```python
from build123d import *

# Parameters (mm, degrees)
SKETCH2_R           = 30
BOSS_EXTRUDE1_DEPTH = 15
SKETCH3_R           = 2.25
CUT_EXTRUDE1_DEPTH  = 9
FILLET1_R           = 1.5
CUT_EXTRUDE2_DEPTH  = 1
SKETCH5_W           = 5
SKETCH5_H           = 19.75
CUT_EXTRUDE3_DEPTH  = 10
CIRPATTERN1_COUNT   = 6


with BuildPart() as part:
    # Sketch2 → Boss-Extrude1 (new body)
    with BuildSketch(Plane(origin=(0, 0, 0), x_dir=(1, 0, 0), z_dir=(0, 1, 0))):
        with Locations(Location((0, 0, 0), (0, 0, 270))):
            Circle(SKETCH2_R)
    extrude(amount=BOSS_EXTRUDE1_DEPTH)

    # Sketch3 → Cut-Extrude1 (cut)
    with BuildSketch(Plane(origin=(0, 15, 0), x_dir=(1, 0, 0), z_dir=(0, 1, 0))):
        with Locations(Location((0, 0, 0), (0, 0, 270))):
            Circle(SKETCH3_R)
    extrude(amount=-CUT_EXTRUDE1_DEPTH, mode=Mode.SUBTRACT)

    # Fillet1
    fillet1_edges = [part.edges().sort_by_distance(p)[0] for p in [
        (0, 0, -30),
        (0, 15, -30),
        (0, 15, -2.25),
    ]]
    fillet(fillet1_edges, radius=FILLET1_R)

    # Sketch4 → Cut-Extrude2 (cut)
    with BuildSketch(Plane.XZ):
        Polygon((-0.5, 24.5), (-0.5, -27.5), (0.5, -27.5), (0.5, 24.5), (3, 24.5), (0, 27.5), (-3, 24.5), align=None)
    extrude(amount=-CUT_EXTRUDE2_DEPTH, mode=Mode.SUBTRACT)

    # Sketch5 → Cut-Extrude3 (cut)
    with BuildSketch(Plane(origin=(0, 15, 0), x_dir=(1, 0, 0), z_dir=(0, 1, 0))):
        with Locations((0, 16.125)):
            Rectangle(SKETCH5_W, SKETCH5_H)
    cut_extrude3 = extrude(amount=-CUT_EXTRUDE3_DEPTH, mode=Mode.SUBTRACT)

    # CirPattern1: Cut-Extrude3 ×6 about axis
    cirpattern1_axis = Axis((0, 0, 0), (0, 1, 0))
    for i in range(1, CIRPATTERN1_COUNT):
        add(cut_extrude3.rotate(cirpattern1_axis, i * 360 / CIRPATTERN1_COUNT), mode=Mode.SUBTRACT)


solid = part.part
```
Part model, mm, in its own coordinate system. Round coordinates to 2 decimals unless told otherwise and drop trailing zeros. Order: outer loops, then holes, each group sorted by start corner. A loop starts at its lowest first (then second) coordinate and runs counter-clockwise, first axis right, second up. Notation, with made-up numbers: M 24.25,-8 L 62.25,-8 A38 cw 62.25,30 Z; hole C 35,38 d8. An arc over 180 degrees is marked long. Put each result on its own line as item: value. Start each with the question number.
1. Slice it at A-A on y = 11.25. List the corners of the cut face in (x, z), then the cut area to 3 significant figures.
2. Slice it at B-B on z = 0. List the corners of the cut face in (x, y).
3. Two-plate mould, pull along X, no slides. Class faces 1 (the face through (-6, 15, 0)), 2 (the face through (2.5, 10, -16)), 3 (the face through (1.32, 7.42, -29.97)), 4 (the face through (-2.5, 10, -16)): +X half, -X half, draft (parallel to the pull), parting line (faces both ways), or undercut.
4. Drill centre lines: probe 1 along X at (y, z) = (9, 0); probe 2 along X at (y, z) = (9.25, -11); probe 3 along Z at (x, y) = (-19.5, 11.75). Where is each one in solid material? Low to high. Write a range as [from, to].
5. Drop flat-ended pins along their axis: pin 1 (4 mm diameter, centred on y = 3, z = 9, fed in from +X); pin 2 (0.5 mm diameter, centred on y = 0.5, z = 5, fed in from -X); pin 3 (1 mm diameter, centred on x = -8.5, y = 13.5, fed in from +Z). Give the stop position or say it passes through.
Findings:
1. outline: C 0,0 d60; hole M -23.77,-10.83 L -21.27,-15.17 L -4.16,-5.29 L -6.66,-0.96 Z; hole M -23.77,10.83 L -6.66,0.96 L -4.16,5.29 L -21.27,15.17 Z; hole M -2.5,-26 L 2.5,-26 L 2.5,-6.25 L -2.5,-6.25 Z; hole M -2.5,6.25 L 2.5,6.25 L 2.5,26 L -2.5,26 Z; hole C 0,0 d4.5; hole M 4.16,-5.29 L 21.27,-15.17 L 23.77,-10.83 L 6.66,-0.96 Z; hole M 4.16,5.29 L 6.66,0.96 L 23.77,10.83 L 21.27,15.17 Z
1. area: 2,220 mm2
2. outline: M -30,1.5 A1.5 ccw -28.5,0 L -0.5,0 L -0.5,1 L 0.5,1 L 0.5,0 L 28.5,0 A1.5 ccw 30,1.5 L 30,13.5 A1.5 ccw 28.5,15 L 3.75,15 A1.5 ccw 2.25,13.5 L 2.25,6 L -2.25,6 L -2.25,13.5 A1.5 ccw -3.75,15 L -28.5,15 A1.5 ccw -30,13.5 Z
3. face 1: draft
3. face 2: undercut
3. face 3: parting line
3. face 4: undercut
4. probe 1: [-30, -2.25], [2.25, 30]
4. probe 2: [-27.91, -23.67], [-14.05, -2.5], [2.5, 14.05], [23.67, 27.91]
4. probe 3: [-22.8, -14.15], [-8.37, 8.37], [14.15, 22.8]
5. pin 1: x = 29.17
5. pin 2: x = -29.38
5. pin 3: z = 28.91
